from build123d import *

# Parameters (mm, degrees)
SKETCH_1_W          = 28.8
SKETCH_1_H          = 16
SKETCH_1_W_2        = 24.8
SKETCH_1_H_2        = 12
EXTRUDE_1_DEPTH     = 16
SKETCH_2_R          = 1.5
CUT_EXTRUDE_1_DEPTH = 28.8
SKETCH_3_R          = 3.7
CUT_EXTRUDE_2_DEPTH = 16
FILLET_1_R          = 4


with BuildPart() as part:
    # 草图1 → 凸台-拉伸1 (new body)
    with BuildSketch(Plane.XY):
        Rectangle(SKETCH_1_W, SKETCH_1_H)
        Rectangle(SKETCH_1_W_2, SKETCH_1_H_2, mode=Mode.SUBTRACT)
    extrude(amount=EXTRUDE_1_DEPTH)

    # 草图2 → 切除-拉伸1 (cut)
    with BuildSketch(Plane(origin=(14.4, 0, 0), x_dir=(0, 0, -1), z_dir=(1, 0, 0))):
        with Locations((-12, 0)):
            Circle(SKETCH_2_R)
        with Locations((-4, 0)):
            Circle(SKETCH_2_R)
    extrude(amount=-CUT_EXTRUDE_1_DEPTH, mode=Mode.SUBTRACT)

    # 草图3 → 切除-拉伸2 (cut)
    with BuildSketch(Plane(origin=(0, 8, 0), x_dir=(1, 0, 0), z_dir=(0, 1, 0))):
        with Locations((0, -8)):
            Circle(SKETCH_3_R)
    extrude(amount=-CUT_EXTRUDE_2_DEPTH, mode=Mode.SUBTRACT)

    # 圆角1
    fillet_1_edges = [part.edges().sort_by_distance(p)[0] for p in [
        (12.4, -6, 8),
        (12.4, 6, 8),
        (-12.4, 6, 8),
        (-12.4, -6, 8),
    ]]
    fillet(fillet_1_edges, radius=FILLET_1_R)


solid = part.part
Geometry: final body of the model. Coordinates: model frame, mm. A direction names the side the tool comes from. Coordinates: 2 decimals unless noted, no trailing zeros. Loops run counter-clockwise (first coordinate to the right, second up) from the corner with the lowest first, then second, coordinate; pieces in that order, holes last. Notation, with made-up numbers: (81, 34.5) - (132, 34.5) arc R3 cw to (132, 38.5) - close; hole circle Ø3 at (68, -28.75). An arc over 180 degrees is marked (long way). Put each result on its own line as item: value. Start each with the question number.
Q1. Pull-direction query (X, two-part tool) for faces 1 (the cylindrical face through (13.41, 0.07, 13.5)), 2 (the cylindrical face through (-0.48, 7.01, 4.33)), 3 (the flat face through (14.4, 0, 8)); classes: released by +X, released by -X, zero draft, split by the parting line, or undercut.
Q2. Set-up query: faces 4 (the flat face through (-3.4, 8, 6.1)), 5 (the flat face through (-4, 6, 8)). Return all of +Z, -Z, +X, -X, +Y, -Y with unobstructed straight access to the full face (end or side cutting, diameter ignored); none if empty.
Q3. Cut plane C-C, the plane y = -4.5. Return loops of the section in (x, z).
Q4. Line query: line 1 (Y direction, x = 4.25, z = 2.75); line 2 (Y direction, x = 13.2, z = 4); line 3 (X direction, y = -0.25, z = 10). Output: solid intervals per line, ascending.
Q5. Cut plane D-D, the plane y = 0. Return loops of the section in (x, z), and give its area (3 significant figures).
Q6. Cut plane B-B, the plane z = 12. Return loops of the section in (x, y), and give its area (3 significant figures).
Q7. Cut plane A-A, the plane x = 0. Return loops of the section in (y, z).
Filled sheet:
1. face 1: zero draft
1. face 2: undercut
1. face 3: released by +X
2. face 4: +Z, -Z, +X, -X, +Y
2. face 5: +Z, -Z
3. outline: (-14.4, 0) - (-11.52, 0) - (-11.52, 16) - (-14.4, 16) - close; (11.52, 0) - (14.4, 0) - (14.4, 16) - (11.52, 16) - close
4. line 1: -8 to -6, 6 to 8
4. line 2: -8 to -1.5, 1.5 to 8
4. line 3: -14.4 to -12.4, 12.4 to 14.4
5. outline: (-14.4, 0) - (-12.4, 0) - (-12.4, 2.5) - (-14.4, 2.5) - close; (-14.4, 5.5) - (-12.4, 5.5) - (-12.4, 10.5) - (-14.4, 10.5) - close; (-14.4, 13.5) - (-12.4, 13.5) - (-12.4, 16) - (-14.4, 16) - close; (12.4, 0) - (14.4, 0) - (14.4, 2.5) - (12.4, 2.5) - close; (12.4, 5.5) - (14.4, 5.5) - (14.4, 10.5) - (12.4, 10.5) - close; (12.4, 13.5) - (14.4, 13.5) - (14.4, 16) - (12.4, 16) - close
5. area: 40.0 mm²
6. outline: (-14.4, -8) - (14.4, -8) - (14.4, -1.5) - (12.4, -1.5) - (12.4, -2) arc R4 cw to (8.4, -6) - (-8.4, -6) arc R4 cw to (-12.4, -2) - (-12.4, -1.5) - (-14.4, -1.5) - close; (-14.4, 1.5) - (-12.4, 1.5) - (-12.4, 2) arc R4 cw to (-8.4, 6) - (8.4, 6) arc R4 cw to (12.4, 2) - (12.4, 1.5) - (14.4, 1.5) - (14.4, 8) - (-14.4, 8) - close
6. area: 165 mm²
7. outline: (-8, 0) - (-6, 0) - (-6, 4.3) - (-8, 4.3) - close; (-8, 11.7) - (-6, 11.7) - (-6, 16) - (-8, 16) - close; (6, 0) - (8, 0) - (8, 4.3) - (6, 4.3) - close; (6, 11.7) - (8, 11.7) - (8, 16) - (6, 16) - close
